Autodesk Inventor part; units mm, degrees
ref_plane "Płaszczyzna konstrukcyjna2" through (0, -80.8223, 0) normal (0, -1, 0) x (1, 0, 0)
ref_plane "YZ Plane" through (0, 0, 0) normal (1, 0, 0) x (0, 1, 0)
ref_plane "XZ Plane" through (0, 0, 0) normal (0, 1, 0) x (-1, 0, 0)
sketch "Szkic6" plane through (0, 0, 0) normal (0, 0, 1) x (1, 0, 0)
  line L0 (-29.6067, 0) -> (35.2678, 0) construction
  line L1 (0, 42.3419) -> (0, -58.3726) construction
  arc A0 (33.4777, 0) -> (0, -80.8223) centre (114.3, -80.8223) ccw
  line L2 (0, -80.8223) -> (114.3, -80.8223) construction
  line L3 (114.3, -80.8223) -> (67.9611, -34.4834) construction
  line L4 (33.4777, 0) -> (63.7892, 30.3115)
  line L5 (0, -80.8223) -> (0, -123.6893)
  point P0 (0, 0)
  dimension "d24" = 114.3
  dimension "d31" = 45
  dimension "d36" = 42.867
  dimension "d37" = 42.867
ref_plane "Płaszczyzna konstrukcyjna2" through (0, -80.8223, 0) normal (0, -1, 0) x (1, 0, 0)
sketch "Szkic8" plane through (0, -80.8223, 0) normal (0, -1, 0) x (1, 0, 0)
  circle A0 centre (0, 0) radius 38.05
  circle A1 centre (0, 0) radius 36.45
  dimension "d32" = 76.1
  dimension "d33" = 1.6
sweep "Przeciągnięcie2" add profiles "Szkic8" path "Szkic6"
equation "\"d32\" = OD"
equation "\"d33\" = THK"
equation "\"d24\" = R"
equation "\"d31\" = KAT"
equation "\"d36\" = PROSTKA"
equation "\"d37\" = PROSTKA"
equation "\"SzerokośćGięciaPodcięcia\" = Grubość"
equation "\"RozmiarPodcięciaNarożnika\" = 4 * Grubość"
equation "\"PromieńPrzejścia\" = PromieńGięcia"
equation "\"Rozmiar_promienia_Jacobiego\" = PromieńGięcia"
equation "\"Wielk_odstępu\" = Grubość"
equation "\"d2\" = PromieńGięcia"
equation "\"d23\" = PromieńGięcia"
equation "\"R\" = 114.3"
equation "\"OD\" = 76.1"
equation "\"THK\" = 1.6"
equation "\"KAT\" = 45deg"
equation "\"PROSTKA\" = 42.867"
properties part number "Kolano 45° ø76,1x1,6 R114,3" material "304L"
Model file for the job. Use its own axes, mm. Give positions to 0.01 mm unless a question says otherwise; leave off trailing zeros. Loops run counter-clockwise (first coordinate to the right, second up) from the corner with the lowest first, then second, coordinate; pieces in that order, holes last. Notation, with made-up numbers: M 6,53 L 44,53 A23 ccw 44,71 Z; hole C -8.5,71 d6. An arc over 180 degrees is marked long. Use one line per item in the form item = value.
Item 1: Drill centre lines: L1, parallel to Z at x = 0, y = -107; L2, parallel to Y at x = 36, z = -28; L3, parallel to Z at x = 20, y = -94. Where is each one in solid material? Low to high.
Filled in:
L1 = -38.05 to -36.45, 36.45 to 38.05
L2 = -39.5 to -34.53, 35.53 to 38.96
L3 = -32.37 to -30.47, 30.47 to 32.37
Item 2: Flat gauge pins, fed straight in: pin 1 Ø10 at (x, z) = (71.5, -13.5) entering from -Y; pin 2 Ø12 at (x, z) = (-6, 19.5) entering from +Y; pin 3 Ø1.5 at (y, z) = (-68.5, 29.5) entering from +X. Where does each tip first touch, or does it go through?
Filled in:
pin_1 = -17.85
pin_2 = 13.14
pin_3 = 25.78
Item 3: Two-plate mould, pull along X, no slides. Class faces 1 (the cylindrical face through (20.46, -102.56, 32.08)), 2 (the flat face through (-31, -123.689, -20)), 3 (the cylindrical face through (34.767, -102.556, 10.949)): released by +X, released by -X, zero draft, split by the parting line, or undercut.
Filled in:
face_1 = split by the parting line
face_2 = zero draft
face_3 = undercut
Item 4: Slice it at A-A on y = -112.5. List the corners of the cut face in (x, z), and give its area (3 significant figures).
Filled in:
outline = C 0,0 d76.1; hole C 0,0 d72.9
area = 374 mm^2
